Build history of the part. All positions in model axes, mm. A direction names the side the tool comes from. Coordinates: 2 decimals unless noted, no trailing zeros. Order: outer loops, then holes, each group sorted by start corner. A loop starts at its lowest first (then second) coordinate and runs counter-clockwise, first axis right, second up. Notation, with made-up numbers: (82.5, 48.25) - (129.5, 48.25) arc R18 ccw to (129.5, 57.25) - close; hole circle Ø11 at (35, 27). An arc over 180 degrees is marked (long way). One line per item, written item: value.
from build123d import *

# Parameters (mm, degrees)
SKETCH1_R           = 73.214752718
BOSS_EXTRUDE4_DEPTH = 20
SKETCH1_7_R         = 16.661107431
SKETCH1_7_R_2       = 10.088971545
CUT_EXTRUDE2_DEPTH  = 20
SKETCH1_8_R         = 29.667707344
CUT_EXTRUDE3_DEPTH  = 10


with BuildPart() as part:
    # Sketch1 → Boss-Extrude4 (new body)
    with BuildSketch(Plane(origin=(0, 0, 0), x_dir=(1, 0, 0), z_dir=(0, 1, 0))):
        with Locations(Location((0, 0, 0), (0, 0, 270))):
            Circle(SKETCH1_R)
    extrude(amount=-BOSS_EXTRUDE4_DEPTH)

    # Sketch1_7 → Cut-Extrude2 (cut)
    with BuildSketch(Plane(origin=(0, 0, 0), x_dir=(1, 0, 0), z_dir=(0, 1, 0))):
        with Locations(Location((0, 0, 0), (0, 0, 270))):
            Circle(SKETCH1_7_R)
        with Locations(Location((-55.576015856, 0, 0), (0, 0, 270))):
            Circle(SKETCH1_7_R_2)
        with Locations(Location((0, 55.576015856, 0), (0, 0, 270))):
            Circle(SKETCH1_7_R_2)
        with Locations(Location((55.576015856, 0, 0), (0, 0, 270))):
            Circle(SKETCH1_7_R_2)
        with Locations(Location((0, -55.576015856, 0), (0, 0, 270))):
            Circle(SKETCH1_7_R_2)
    extrude(amount=-CUT_EXTRUDE2_DEPTH, mode=Mode.SUBTRACT)

    # Sketch1_8 → Cut-Extrude3 (cut)
    with BuildSketch(Plane(origin=(0, 0, 0), x_dir=(1, 0, 0), z_dir=(0, 1, 0))):
        with BuildLine():
            ThreePointArc((52.703821385, -17.635213348), (37.708440449, 0), (52.703821385, 17.635213348))
            ThreePointArc((52.703821385, 17.635213348), (39.298177683, 39.298177683), (17.635213348, 52.703821385))
            ThreePointArc((17.635213348, 52.703821385), (0, 37.708440449), (-17.635213348, 52.703821385))
            ThreePointArc((-17.635213348, 52.703821385), (-39.298177683, 39.298177683), (-52.703821385, 17.635213348))
            ThreePointArc((-52.703821385, 17.635213348), (-41.96408355, 11.574348786), (-37.708440449, 0))
            ThreePointArc((-37.708440449, 0), (-41.96408355, -11.574348786), (-52.703821385, -17.635213348))
            ThreePointArc((-52.703821385, -17.635213348), (-39.298177683, -39.298177683), (-17.635213348, -52.703821385))
            ThreePointArc((-17.635213348, -52.703821385), (0, -37.708440449), (17.635213348, -52.703821385))
            ThreePointArc((17.635213348, -52.703821385), (39.298177683, -39.298177683), (52.703821385, -17.635213348))
        make_face()
        with Locations(Location((0, 0, 0), (0, 0, 270))):
            Circle(SKETCH1_8_R, mode=Mode.SUBTRACT)
    extrude(amount=-CUT_EXTRUDE3_DEPTH, mode=Mode.SUBTRACT)


solid = part.part
1. Band-saw the part on D-D, the plane z = -59. Give the cut face in (x, y), and give its area (3 significant figures).
Values found:
outline: (-43.35, -20) - (-9.49, -20) - (-9.49, 0) - (-43.35, 0) - close; (9.49, -20) - (43.35, -20) - (43.35, 0) - (9.49, 0) - close
area: 1,350 mm2
2. Band-saw the part on C-C, the plane x = -48. Give the cut face in (y, z).
Values found:
outline: (-20, -55.28) - (0, -55.28) - (0, -28.01) - (-10, -28.01) - (-10, -16.18) - (0, -16.18) - (0, -6.66) - (-20, -6.66) - close; (-20, 6.66) - (0, 6.66) - (0, 16.18) - (-10, 16.18) - (-10, 28.01) - (0, 28.01) - (0, 55.28) - (-20, 55.28) - close
3. 3-axis set-ups, long thin cutter, end or side, ignore diameter. For faces 1 (the face through (29.415, -4.93, -3.862)), 2 (the face through (-65.425, -9.86, -2.187)): which of +Z, -Z, +X, -X, +Y, -Y reach the whole face in a straight line?
Values found:
face 1: +Y
face 2: +Y, -Y
4. Two-plate mould, pull along X, no slides. Class faces 3 (the face through (-48, 0, 15)), 4 (the face through (0.444, -9.86, -65.655)), 5 (the face through (72.59, -9.86, -9.53)): pulls with the +X half, pulls with the -X half, needs draft (parallel to the pull), parting line crosses it, or undercut.
Values found:
face 3: needs draft
face 4: undercut
face 5: parting line crosses it
5. Flat gauge pins, fed straight in: P1, Ø1.5, axis at x = -43.5, y = -5.5, coming from the +Z side; P2, Ø12, axis at x = -36, y = -17.5, coming from the -Z side; P3, Ø8, axis at x = -28.5, y = -13, coming from the +Z side. Where does each tip first touch, or does it go through?
Values found:
P1: stops at z = 59.44
P2: stops at z = -66.79
P3: stops at z = 68.99
6. Band-saw the part on A-A, the plane x = 0. Give the cut face in (y, z), and give its area (3 significant figures).
Values found:
outline: (-20, -73.21) - (0, -73.21) - (0, -65.66) - (-20, -65.66) - close; (-20, -45.49) - (0, -45.49) - (0, -37.71) - (-10, -37.71) - (-10, -29.67) - (0, -29.67) - (0, -16.66) - (-20, -16.66) - close; (-20, 16.66) - (0, 16.66) - (0, 29.67) - (-10, 29.67) - (-10, 37.71) - (0, 37.71) - (0, 45.49) - (-20, 45.49) - close; (-20, 65.66) - (0, 65.66) - (0, 73.21) - (-20, 73.21) - close
area: 1,290 mm2
7. Band-saw the part on B-B, the plane y = -3. Give the cut face in (x, z).
Values found:
outline: circle Ø146.43 at (0, 0); circle Ø59.34 at (0, 0); hole circle Ø20.18 at (-55.58, 0); hole (-52.7, -17.64) arc R55.58 ccw to (-17.64, -52.7) arc R17.87 cw to (17.64, -52.7) arc R55.58 ccw to (52.7, -17.64) arc R17.87 cw to (52.7, 17.64) arc R55.58 ccw to (17.64, 52.7) arc R17.87 cw to (-17.64, 52.7) arc R55.58 ccw to (-52.7, 17.64) arc R17.87 cw to start; hole circle Ø33.32 at (0, 0); hole circle Ø20.18 at (0, -55.58); hole circle Ø20.18 at (0, 55.58); hole circle Ø20.18 at (55.58, 0)
8. Probe line 1 along X through (y, z) = (-11.5, 0); line 2 along Z through (x, y) = (0.5, -17); line 3 along X through (y, z) = (-3.5, 25). List the from-to ranges inside material, lowest first.
Values found:
line 1: x = -73.21 to -65.66, -45.49 to -16.66, 16.66 to 45.49, 65.66 to 73.21
line 2: z = -73.21 to -65.65, -45.5 to -16.65, 16.65 to 45.5, 65.65 to 73.21
line 3: x = -68.81 to -49.64, -15.97 to 15.97, 49.64 to 68.81
